Autodesk Inventor part; units mm, degrees
ref_plane "YZ Plane" through (0, 0, 0) normal (1, 0, 0) x (0, 1, 0)
ref_plane "XZ Plane" through (0, 0, 0) normal (0, 1, 0) x (-1, 0, 0)
ref_plane "XY Plane" through (0, 0, 0) normal (0, 0, 1) x (1, 0, 0)
sketch "Skizze2" plane through (0, 0, 0) normal (0, 0, 1) x (1, 0, 0)
  line L0 (47.429, 1.628) -> (41.9536, 1.5965)
  line L1 (47.4645, -1.7719) -> (41.9641, -1.8346)
  line L2 (41.9168, 1.5642) -> (41.9437, -0.1365)
  line L3 (47.466, 0.6928) -> (47.4706, 0.1306)
  line L4 (48.1143, -2.2865) -> (41.3143, -2.2865)
  line L5 (41.3143, -2.2865) -> (41.3143, 2.0135)
  line L6 (41.3143, 2.0135) -> (48.1143, 2.0135)
  line L7 (48.1143, 2.0135) -> (48.1143, -2.2865)
  line L8 (48.1143, -2.2865) -> (41.3143, 2.0135) construction
  line L9 (41.3143, -2.2865) -> (48.1143, 2.0135) construction
  point P0 (0, 0)
  point P1 (44.7143, -0.1365)
  dimension "d0" = 6.8
  dimension "d1" = 4.3
extrude "Extrusion1" add sketch "Skizze2" against normal blind 6
sketch "Skizze4" plane through (0, 0, -6) normal (0, 0, -1) x (-1, 0, 0)
  line L0 (-48.1143, -2.2865) -> (-41.3143, -2.2865) construction
  line L1 (-41.3143, 2.0135) -> (-48.1143, 2.0135) construction
  line L2 (-41.3143, -2.2865) -> (-41.3143, 2.0135) construction
  line L3 (-48.1143, 2.0135) -> (-48.1143, -2.2865) construction
  line L4 (-49.8143, -10.2365) -> (-39.6143, -10.2365)
  line L5 (-39.6143, -10.2365) -> (-39.6143, 9.9635)
  line L6 (-39.6143, 9.9635) -> (-49.8143, 9.9635)
  line L7 (-49.8143, -10.2365) -> (-39.6143, 9.9635) construction
  line L8 (-39.6143, -10.2365) -> (-49.8143, 9.9635) construction
  line L9 (-59.8143, -5.2365) -> (-59.8143, 4.9635)
  line L10 (-29.6143, -5.2365) -> (-59.8143, 4.9635) construction
  line L11 (-59.8143, -5.2365) -> (-29.6143, 4.9635) construction
  line L12 (-41.3143, -5.2365) -> (-42.1391, -5.2365)
  line L13 (-49.8143, -5.2365) -> (-59.8143, -5.2365)
  line L14 (-59.8143, 4.9635) -> (-49.8143, 4.9635)
  line L15 (-42.1391, 4.9635) -> (-41.3143, 4.9635)
  line L16 (-49.8143, 9.9635) -> (-49.8143, 4.9635)
  line L17 (-49.8143, -5.2365) -> (-49.8143, -10.2365)
  point P0 (0, 0)
  point P1 (-44.7143, -0.1365)
  point P2 (-44.7143, -0.1365)
extrude "Extrusion2" add sketch "Skizze4" along normal blind 2
fillet "Rundung1" radius 1 4 edges at (44.7143, 2.0135, 0) (41.3143, -0.1365, 0) (48.1143, -0.1365, 0) (44.7143, -2.2865, 0)
sketch "Skizze5" plane through (0, 0, 0) normal (0, 0, 1) x (1, 0, 0)
  line L0 (49.8143, -10.2365) -> (39.6143, -10.2365)
  line L1 (49.8143, -5.2365) -> (49.8143, -10.2365)
  line L2 (59.8143, -5.2365) -> (49.8143, -5.2365)
  line L3 (59.8143, 4.9635) -> (59.8143, -5.2365)
  line L4 (49.8143, 4.9635) -> (59.8143, 4.9635)
  line L5 (49.8143, 9.9635) -> (49.8143, 4.9635)
  line L6 (39.6143, 9.9635) -> (49.8143, 9.9635)
  line L7 (39.6143, -10.2365) -> (39.6143, 9.9635)
  line L8 (48.1143, 2.0135) -> (48.1143, -2.2865)
  line L9 (48.1143, -2.2865) -> (41.3143, -2.2865)
  line L10 (41.3143, -2.2865) -> (41.3143, 2.0135)
  line L11 (41.3143, 2.0135) -> (48.1143, 2.0135)
  point P0 (0, 0)
extrude "Extrusion3" cut sketch "Skizze5" against normal blind 2 contours L8 L9 L10 L11
fillet "Rundung2" radius 0.5 4 edges at (44.7143, 2.0135, -2) (41.3143, -0.1365, -2) (44.7143, -2.2865, -2) (48.1143, -0.1365, -2)
sketch "Skizze6" plane through (0, 0, -8) normal (0, 0, -1) x (-1, 0, 0)
  line L0 (-49.8143, -10.2365) -> (-39.6143, -10.2365)
  line L1 (-39.6143, -10.2365) -> (-39.6143, 9.9635)
  line L2 (-39.6143, 9.9635) -> (-49.8143, 9.9635)
  line L3 (-49.8143, 9.9635) -> (-49.8143, 4.9635)
  line L4 (-49.8143, 4.9635) -> (-59.8143, 4.9635)
  line L5 (-59.8143, 4.9635) -> (-59.8143, -5.2365)
  line L6 (-59.8143, -5.2365) -> (-49.8143, -5.2365)
  line L7 (-49.8143, -5.2365) -> (-49.8143, -10.2365)
  line L8 (-39.6143, -10.2365) -> (-39.6143, 9.9635)
  line L9 (-39.6143, 4.9635) -> (-29.6143, 4.9635)
  line L10 (-29.6143, 4.9635) -> (-29.6143, -5.2365)
  line L11 (-29.6143, -5.2365) -> (-39.6143, -5.2365)
  line L12 (-39.6143, -5.2365) -> (-39.6143, 4.9635)
  point P0 (0, 0)
  dimension "d14" = 10
extrude "Extrusion4" add sketch "Skizze6" against normal up to surface (2 mm away) contours L1 L9 L10 L11
properties part number "palm_plate" material "Nylon 6/6"
Design review of the part built by this model. Coordinates are the model's own, in mm. A direction names the side the tool comes from. Give positions to 0.01 mm unless a question says otherwise; leave off trailing zeros. Order: outer loops, then holes, each group sorted by start corner. A loop starts at its lowest first (then second) coordinate and runs counter-clockwise, first axis right, second up. Notation, with made-up numbers: M 16,-32 L 59,-32 A23 ccw 59,-8 Z; hole C 80,2.25 d5. An arc over 180 degrees is marked long. One line per question, with ' | ' between items. Start each with the question number.
Q1. We need section A-A (z = -6.9). Write out the cut boundary in (x, y), plus the area to 3 significant figures.
Q2. For L1, parallel to Z at x = 42.5, y = -5.5; L2, parallel to X at y = 9, z = -6.3; L3, parallel to Y at x = 42, z = -2.5, list the stretches that pass through material, from the lowest coordinate up. Write a range as [from, to].
Q3. We need section D-D (x = 41). Write out the cut boundary in (y, z).
Q4. Machinability: for faces 1 (the face through (41.314, 0, -4)), 2 (the face through (55, -5.236, -7)), 3 (the face through (39.614, -8, -7)), 4 (the face through (39.614, 7, -7)), 5 (the face through (48.114, 0, -4)), which of the approach directions +Z, -Z, +X, -X, +Y, -Y give a long, thin tool a straight path to every point of the face, cutting with its end or side? Answer none if there is none.
Q5. For pin 1 Ø1 at (x, z) = (32.5, -7) entering from +Y; pin 2 Ø2 at (x, z) = (33, -6.5) entering from -Y; pin 3 Ø1 at (y, z) = (0.5, -4) entering from -X, all flat-tipped, find the tip position at first contact; note any pin that passes through.
Q6. We need section C-C (y = -3.5). Write out the cut boundary in (x, z).
Q7. We need section B-B (x = 45). Write out the cut boundary in (y, z).
Returned:
1) outline: M 29.61,-5.24 L 39.61,-5.24 L 39.61,-10.24 L 49.81,-10.24 L 49.81,-5.24 L 59.81,-5.24 L 59.81,4.96 L 49.81,4.96 L 49.81,9.96 L 39.61,9.96 L 39.61,4.96 L 29.61,4.96 Z | area: 410 mm2
2) L1: [-8, -6] | L2: [39.61, 49.81] | L3: [-2.29, 2.01]
3) outline: M -10.24,-8 L 9.96,-8 L 9.96,-6 L -10.24,-6 Z
4) face 1: +Z, -X, +Y, -Y | face 2: +Z, -Z, +X, -Y | face 3: +Z, -Z, -X, -Y | face 4: +Z, -Z, -X, +Y | face 5: +Z, +X, +Y, -Y
5) pin 1: y = 4.96 | pin 2: y = -5.24 | pin 3: x = 41.31
6) outline: M 29.61,-8 L 59.81,-8 L 59.81,-6 L 29.61,-6 Z
7) outline: M -10.24,-8 L 9.96,-8 L 9.96,-6 L 2.01,-6 L 2.01,-2.5 A0.5 ccw 1.51,-2 L -1.79,-2 A0.5 ccw -2.29,-2.5 L -2.29,-6 L -10.24,-6 Z
